```python
from build123d import *

# Parameters (mm, degrees)
SKETCH1_W                      = 508
SKETCH1_H                      = 63.5
BASE_FLANGE1_DEPTH             = 3.175
EDGE_FLANGE1_STRIP_W           = 22.2504
EDGE_FLANGE1_STRIP_H           = 3.175
EDGE_FLANGE1_STRIP_CUT_DEPTH   = 508
EDGE_FLANGE1_STRIP_2_W         = 22.2504
EDGE_FLANGE1_STRIP_2_H         = 3.175
EDGE_FLANGE1_STRIP_CUT_2_DEPTH = 508
EDGE_FLANGE1_DEPTH             = 508
EDGE_FLANGE1_BEND_DEPTH        = 508
SKETCH12_R                     = 12.7
CUT_EXTRUDE1_DEPTH             = 277.498571425
SKETCH13_R                     = 6.35
CUT_EXTRUDE2_DEPTH             = 277.498571425
CUT_EXTRUDE4_DEPTH             = 277.498571425
SKETCH16_R                     = 6.35
CUT_EXTRUDE5_DEPTH             = 277.498571425
CUT_EXTRUDE6_DEPTH             = 277.498571425
SKETCH18_R                     = 6.35
CUT_EXTRUDE8_DEPTH             = 277.498571425
SKETCH22_W                     = 19.05
SKETCH22_H                     = 50.682224045
CUT_EXTRUDE9_DEPTH             = 277.498571425
EDGE_FLANGE2_STRIP_W           = 22.2504
EDGE_FLANGE2_STRIP_H           = 3.175
EDGE_FLANGE2_STRIP_CUT_DEPTH   = 88.9
EDGE_FLANGE2_RELIEF_W          = 23.8379
EDGE_FLANGE2_RELIEF_H          = 1.5875
EDGE_FLANGE2_RELIEF_CUT_DEPTH  = 3.175
EDGE_FLANGE2_DEPTH             = 88.9


# Sheet-metal steps are written as plain solids
with BuildPart() as part:
    # Sketch1 → Base-Flange1 (new body)
    with BuildSketch(Plane(origin=(0, 0, 0), x_dir=(1, 0, 0), z_dir=(0, 1, 0))):
        Rectangle(SKETCH1_W, SKETCH1_H)
    extrude(amount=-BASE_FLANGE1_DEPTH)

    # Edge-Flange1 strip (across the edge) → Edge-Flange1 strip cut (cut)
    with BuildSketch(Plane(origin=(254, -3.175, 31.75), x_dir=(0, 0, -1), z_dir=(-1, 0, 0))):
        with Locations((-3.175, -1.5875)):
            Rectangle(EDGE_FLANGE1_STRIP_W, EDGE_FLANGE1_STRIP_H)
    extrude(amount=EDGE_FLANGE1_STRIP_CUT_DEPTH, mode=Mode.SUBTRACT)

    # Edge-Flange1 strip 2 (across the edge) → Edge-Flange1 strip cut 2 (cut)
    with BuildSketch(Plane(origin=(-254, -3.175, -31.75), x_dir=(0, 0, 1), z_dir=(1, 0, 0))):
        with Locations((-3.175, -1.5875)):
            Rectangle(EDGE_FLANGE1_STRIP_2_W, EDGE_FLANGE1_STRIP_2_H)
    extrude(amount=EDGE_FLANGE1_STRIP_CUT_2_DEPTH, mode=Mode.SUBTRACT)

    # Edge-Flange1 section (across the edge) → Edge-Flange1 (add)
    with BuildSketch(Plane(origin=(254, -3.175, 31.75), x_dir=(0, 0, -1), z_dir=(-1, 0, 0))):
        with BuildLine():
            Line((0, 4.7752), (0, 85.725))
            Line((0, 85.725), (3.175, 85.725))
            Line((3.175, 85.725), (3.175, 4.7752))
            ThreePointArc((3.175, 4.7752), (4.573623698, 1.398623698), (7.9502, 0))
            Line((7.9502, 0), (7.9502, -3.175))
            ThreePointArc((7.9502, -3.175), (2.328559668, -0.846440332), (0, 4.7752))
        make_face()
    extrude(amount=EDGE_FLANGE1_DEPTH)

    # Edge-Flange1 section 2 (across the edge) → Edge-Flange1 bend (add)
    with BuildSketch(Plane(origin=(-254, -3.175, -31.75), x_dir=(0, 0, 1), z_dir=(1, 0, 0))):
        with BuildLine():
            Line((0, 4.7752), (0, 85.725))
            Line((0, 85.725), (3.175, 85.725))
            Line((3.175, 85.725), (3.175, 4.7752))
            ThreePointArc((3.175, 4.7752), (4.573623698, 1.398623698), (7.9502, 0))
            Line((7.9502, 0), (7.9502, -3.175))
            ThreePointArc((7.9502, -3.175), (2.328559668, -0.846440332), (0, 4.7752))
        make_face()
    extrude(amount=EDGE_FLANGE1_BEND_DEPTH)

    # Sketch12 → Cut-Extrude1 (cut, through all)
    with BuildSketch(Plane.XY.offset(31.75)):
        with Locations((0, -33.02)):
            Circle(SKETCH12_R)
    extrude(amount=-CUT_EXTRUDE1_DEPTH, mode=Mode.SUBTRACT)

    # Sketch13 → Cut-Extrude2 (cut, through all)
    with BuildSketch(Plane.XY.offset(31.75)):
        with Locations((88.9, -54.166128078)):
            Circle(SKETCH13_R)
    extrude(amount=-CUT_EXTRUDE2_DEPTH, mode=Mode.SUBTRACT)

    # Sketch14 → Cut-Extrude4 (cut, through all)
    with BuildSketch(Plane.XY.offset(31.75)):
        with BuildLine():
            Line((-65.991135768, -50.8), (-203.2, -50.8))
            ThreePointArc((-203.2, -50.8), (-228.6, -76.2), (-254, -50.8))
            Line((-254, -50.8), (-254, -88.9))
            Line((-254, -88.9), (0, -88.9))
            Line((0, -88.9), (-65.991135768, -50.8))
        make_face()
    extrude(amount=-CUT_EXTRUDE4_DEPTH, mode=Mode.SUBTRACT)

    # Sketch16 → Cut-Extrude5 (cut, through all)
    with BuildSketch(Plane.XY.offset(31.75)):
        with Locations((-228.6, -50.8)):
            Circle(SKETCH16_R)
    extrude(amount=-CUT_EXTRUDE5_DEPTH, mode=Mode.SUBTRACT)

    # Sketch17 → Cut-Extrude6 (cut, through all)
    with BuildSketch(Plane.XY.offset(31.75)):
        with BuildLine():
            ThreePointArc((254, -46.0375), (250.338556711, -59.209109907), (240.404769023, -68.601518366))
            Line((240.404769023, -68.601518366), (202.003688132, -88.9))
            Line((202.003688132, -88.9), (254, -88.9))
            Line((254, -88.9), (254, -46.0375))
        make_face()
    extrude(amount=-CUT_EXTRUDE6_DEPTH, mode=Mode.SUBTRACT)

    # Sketch18 → Cut-Extrude8 (cut, through all)
    with BuildSketch(Plane.XY.offset(31.75)):
        with Locations((228.477622657, -46.0375)):
            Circle(SKETCH18_R)
    extrude(amount=-CUT_EXTRUDE8_DEPTH, mode=Mode.SUBTRACT)

    # Sketch22 → Cut-Extrude9 (cut, through all)
    with BuildSketch(Plane.XY.offset(31.75)):
        with Locations((149.225, -25.341112023)):
            Rectangle(SKETCH22_W, SKETCH22_H)
    extrude(amount=-CUT_EXTRUDE9_DEPTH, mode=Mode.SUBTRACT)

    # Edge-Flange2 strip (across the edge) → Edge-Flange2 strip cut (cut)
    with BuildSketch(Plane(origin=(133.35, -88.9, -31.75), x_dir=(0, 1, 0), z_dir=(-1, 0, 0))):
        with Locations((-3.175, -1.5875)):
            Rectangle(EDGE_FLANGE2_STRIP_W, EDGE_FLANGE2_STRIP_H)
    edge_flange2_strip_cut = extrude(amount=EDGE_FLANGE2_STRIP_CUT_DEPTH, mode=Mode.SUBTRACT)

    # Edge-Flange2 relief (on the sheet) → Edge-Flange2 relief cut (cut)
    with BuildSketch(Plane(origin=(133.35, -80.9498, -31.75), x_dir=(0, 1, 0), z_dir=(0, 0, -1))):
        with Locations((-10.33145, 0.79375)):
            Rectangle(EDGE_FLANGE2_RELIEF_W, EDGE_FLANGE2_RELIEF_H)
        with Locations((-10.33145, -89.69375)):
            Rectangle(EDGE_FLANGE2_RELIEF_W, EDGE_FLANGE2_RELIEF_H)
    edge_flange2_relief_cut = extrude(amount=-EDGE_FLANGE2_RELIEF_CUT_DEPTH, mode=Mode.SUBTRACT)

    # Edge-Flange2 section (across the edge) → Edge-Flange2 (add)
    with BuildSketch(Plane(origin=(133.35, -88.9, -31.75), x_dir=(0, 1, 0), z_dir=(-1, 0, 0))):
        with BuildLine():
            Line((0, 4.7752), (0, 22.225))
            Line((0, 22.225), (3.175, 22.225))
            Line((3.175, 22.225), (3.175, 4.7752))
            ThreePointArc((3.175, 4.7752), (4.573623698, 1.398623698), (7.9502, 0))
            Line((7.9502, 0), (7.9502, -3.175))
            ThreePointArc((7.9502, -3.175), (2.328559668, -0.846440332), (0, 4.7752))
        make_face()
    edge_flange2 = extrude(amount=EDGE_FLANGE2_DEPTH)

    # Mirror1: Edge-Flange2 strip cut, Edge-Flange2 relief cut, Edge-Flange2 across plane
    add(edge_flange2_strip_cut.mirror(Plane.XY), mode=Mode.SUBTRACT)
    add(edge_flange2_relief_cut.mirror(Plane.XY), mode=Mode.SUBTRACT)
    add(edge_flange2.mirror(Plane.XY))


solid = part.part
```
Design review of the part built by this model. Coordinates are the model's own, in mm. A direction names the side the tool comes from. Coordinates: 2 decimals unless noted, no trailing zeros. Order: outer loops, then holes, each group sorted by start corner. A loop starts at its lowest first (then second) coordinate and runs counter-clockwise, first axis right, second up. Notation, with made-up numbers: (57.25, -10.5) -> (66.25, -10.5) arc R28 ccw to (66.25, 10.5) -> close; hole circle Ø1 at (83.25, -23.75). An arc over 180 degrees is marked (long way). One line per item, written item: value. Start each with the question number.
Q1. Insertion check: pin 1 Ø0.5 at (x, z) = (134, -30) entering from -Y; pin 2 Ø6 at (x, y) = (-34.5, -34.5) entering from +Z; pin 3 Ø14 at (x, z) = (98.5, 44) entering from +Y (3 decimals). Each pin has a flat end and moves straight along its axis. Give the tip position at first contact, or say it passes through.
Q2. Tool access review of faces 5 (the flat face through (-4, -49, -28.575)), 6 (the flat face through (44.45, -86, 41)), 7 (the flat face through (158.75, -3, 0)): name each direction out of +Z, -Z, +X, -X, +Y, -Y from which nothing blocks a thin tool from reaching the whole face with its end or side.
Q3. Take a section at C-C, the plane x = -228.6. State the section outline as (y, z) points (3 decimals), then the cut area to 3 significant figures.
Q4. Take a section at D-D, the plane z = 4. State the section outline as (x, y) points (3 decimals), then the cut area to 3 significant figures.
Q5. Take a section at B-B, the plane y = -33.02. State the section outline as (x, z) points (3 decimals), then the cut area to 3 significant figures.
Q6. For probe 1 along Z at (x, y) = (-81.5, -37) (3 decimals); probe 2 along Y at (x, z) = (129, -44) (3 decimals); probe 3 along X at (y, z) = (-84, -31.5), list the stretches that pass through material, from the lowest coordinate up.
Q7. Take a section at A-A, the plane y = -14. State the section outline as (x, z) points (3 decimals), then the cut area to 3 significant figures.
Q8. Mouldability with a two-part tool opening along Y and no side actions: class faces 1 (the cylindrical face through (234.534, -44.13, 30.185)), 2 (the flat face through (44.45, -86, -41)), 3 (the cylindrical face through (-234.944, -50.521, -30.14)), 4 (the flat face through (90, -85.725, -45)) as pulls with the +Y half, pulls with the -Y half, needs draft (parallel to the pull), parting line crosses it, or undercut.
Values follow:
1. pin 1: stops at y = -79.36
1. pin 2: stops at z = 31.75
1. pin 3: stops at y = -85.725
2. face 5: +X, -X, -Y
2. face 6: +Z, -Z, -Y
2. face 7: +Z, -Z, +Y
3. outline: (-76.2, -31.75) -> (-57.15, -31.75) -> (-57.15, -28.575) -> (-76.2, -28.575) -> close; (-76.2, 28.575) -> (-57.15, 28.575) -> (-57.15, 31.75) -> (-76.2, 31.75) -> close; (-44.45, -31.75) -> (-7.95, -31.75) arc R7.95 ccw to (0, -23.8) -> (0, 23.8) arc R7.95 ccw to (-7.95, 31.75) -> (-44.45, 31.75) -> (-44.45, 28.575) -> (-7.95, 28.575) arc R4.775 cw to (-3.175, 23.8) -> (-3.175, -23.8) arc R4.775 cw to (-7.95, -28.575) -> (-44.45, -28.575) -> close
3. area: 567 mm2
4. outline: (-254, -3.175) -> (139.7, -3.175) -> (139.7, 0) -> (-254, 0) -> close; (158.75, -3.175) -> (254, -3.175) -> (254, 0) -> (158.75, 0) -> close
4. area: 1,550 mm2
5. outline: (-254, -31.75) -> (-12.7, -31.75) -> (-12.7, -28.575) -> (-254, -28.575) -> close; (-254, 28.575) -> (-12.7, 28.575) -> (-12.7, 31.75) -> (-254, 31.75) -> close; (12.7, -31.75) -> (139.7, -31.75) -> (139.7, -28.575) -> (12.7, -28.575) -> close; (12.7, 28.575) -> (139.7, 28.575) -> (139.7, 31.75) -> (12.7, 31.75) -> close; (158.75, -31.75) -> (254, -31.75) -> (254, -28.575) -> (158.75, -28.575) -> close; (158.75, 28.575) -> (254, 28.575) -> (254, 31.75) -> (158.75, 31.75) -> close
5. area: 2,940 mm2
6. probe 1: z = -31.75 to -28.575, 28.575 to 31.75
6. probe 2: y = -88.9 to -85.725
6. probe 3: x = -8.49 to 42.86, 44.45 to 133.35, 134.94 to 211.27
7. outline: (-254, -31.75) -> (139.7, -31.75) -> (139.7, -28.575) -> (-254, -28.575) -> close; (-254, 28.575) -> (139.7, 28.575) -> (139.7, 31.75) -> (-254, 31.75) -> close; (158.75, -31.75) -> (254, -31.75) -> (254, -28.575) -> (158.75, -28.575) -> close; (158.75, 28.575) -> (254, 28.575) -> (254, 31.75) -> (158.75, 31.75) -> close
7. area: 3,100 mm2
8. face 1: undercut
8. face 2: needs draft
8. face 3: undercut
8. face 4: pulls with the +Y half
